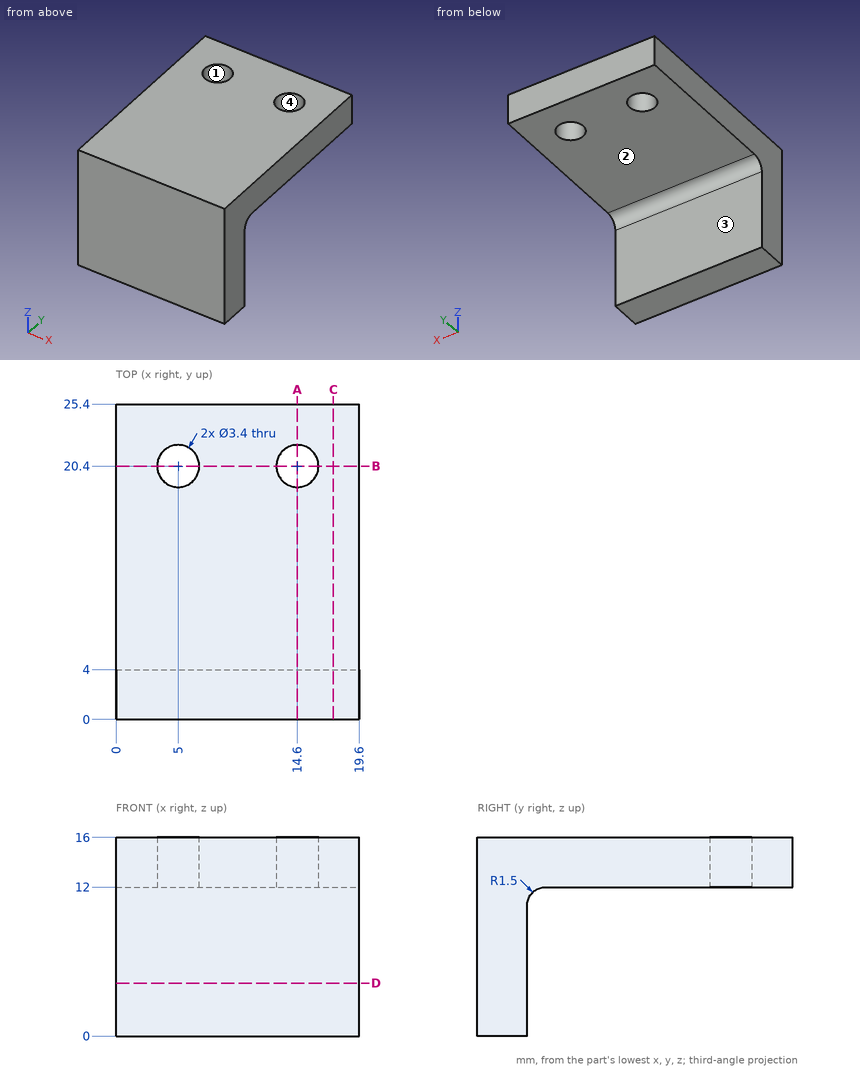
Answer from the drawing. Dimensions are ordinates in mm from the lowest x, y and z of the part. Coordinates: 2 decimals unless noted, no trailing zeros. Order: outer loops, then holes, each group sorted by start corner. A loop starts at its lowest first (then second) coordinate and runs counter-clockwise, first axis right, second up. Notation, with made-up numbers: (80.5, -7.5) - (86.5, -7.5) arc R23 ccw to (86.5, 5.5) - close; hole circle Ø2 at (72, 36.25). An arc over 180 degrees is marked (long way). Use one line per item in the form item = value.
(1) Section B-B, the plane y = 20.4 is taken. Give the vertices of the cut face in (x, z).
Computed values:
outline = (0, 12) - (3.3, 12) - (3.3, 16) - (0, 16) - close; (6.7, 12) - (12.9, 12) - (12.9, 16) - (6.7, 16) - close; (16.3, 12) - (19.6, 12) - (19.6, 16) - (16.3, 16) - close
(2) Given pin 1 Ø5 at (x, z) = (17, 9) entering from +Y; pin 2 Ø2 at (x, z) = (10, 4) entering from +Y; pin 3 Ø4 at (x, y) = (17.5, 21.5) entering from -Z; pin 4 Ø2 at (x, y) = (14.6, 20.4) entering from +Z, each flat-ended and moving along its own axis, determine where each tip first touches the part or whether it passes through.
Computed values:
pin_1 = 4.38
pin_2 = 4
pin_3 = 12
pin_4 = through
(3) Straight lines are drawn through the part: L1, parallel to Y at x = 14.6, z = 13.45; L2, parallel to Z at x = 14, y = 16; L3, parallel to Y at x = 9.5, z = 10. For each, find the intervals that lie inside material, in ascending order.
Computed values:
L1 = 0 to 18.7, 22.1 to 25.4
L2 = 12 to 16
L3 = 0 to 4
(4) Section C-C, the plane x = 17.5 is taken. Give the vertices of the cut face in (y, z), then the cut area to 3 significant figures.
Computed values:
outline = (0, 0) - (4, 0) - (4, 10.5) arc R1.5 cw to (5.5, 12) - (25.4, 12) - (25.4, 16) - (0, 16) - close
area = 150 mm²
(5) For a pull along Y with two mould halves and no side action, classify the marked faces 1, 2, 3 and 4 as pulls with the +Y half, pulls with the -Y half, needs draft (parallel to the pull), parting line crosses it, or undercut.
Computed values:
face_1 = undercut
face_2 = needs draft
face_3 = pulls with the +Y half
face_4 = undercut
(6) Section D-D, the plane z = 4.25 is taken. Give the vertices of the cut face in (x, y).
Computed values:
outline = (0, 0) - (19.6, 0) - (19.6, 4) - (0, 4) - close
(7) Section A-A, the plane x = 14.6 is taken. Give the vertices of the cut face in (y, z).
Computed values:
outline = (0, 0) - (4, 0) - (4, 10.5) arc R1.5 cw to (5.5, 12) - (18.7, 12) - (18.7, 16) - (0, 16) - close; (22.1, 12) - (25.4, 12) - (25.4, 16) - (22.1, 16) - close
